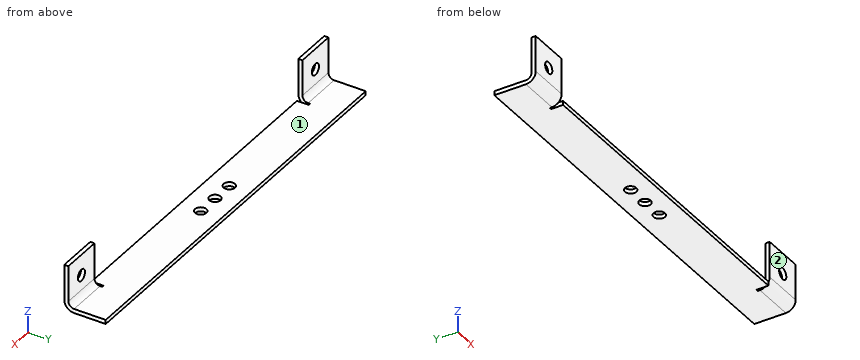
```python
from build123d import *

# Parameters (mm, degrees)
SKETCH_1_W                        = 200
SKETCH_1_H                        = 20
SM_BASE_FLANGE_1_DEPTH            = 2
SM_EDGE_FLANGE_1_STRIP_W          = 13.4732
SM_EDGE_FLANGE_1_STRIP_H          = 2
SM_EDGE_FLANGE_1_STRIP_CUT_DEPTH  = 20
SM_EDGE_FLANGE_1_RELIEF_W         = 14.4732
SM_EDGE_FLANGE_1_RELIEF_H         = 1
SM_EDGE_FLANGE_1_RELIEF_CUT_DEPTH = 2
SM_EDGE_FLANGE_1_DEPTH            = 20
SKETCH_10_R                       = 2.75
CUT_EXTRUDE_2_DEPTH               = 10
SKETCH_11_R                       = 2.75
CUT_EXTRUDE_3_DEPTH               = 10


# Sheet-metal steps are written as plain solids
with BuildPart() as part:
    # Sketch 1 → 基体-法兰1 (new body)
    with BuildSketch(Plane.XY):
        with Locations((0, -10)):
            Rectangle(SKETCH_1_W, SKETCH_1_H)
    extrude(amount=-SM_BASE_FLANGE_1_DEPTH)

    # 边线-法兰1 strip (across the edge) → 边线-法兰1 strip cut (cut)
    with BuildSketch(Plane(origin=(-100, -20, 0), x_dir=(0, 1, 0), z_dir=(1, 0, 0))):
        with Locations((-2, -1)):
            Rectangle(SM_EDGE_FLANGE_1_STRIP_W, SM_EDGE_FLANGE_1_STRIP_H)
    sm_edge_flange_1_strip_cut = extrude(amount=SM_EDGE_FLANGE_1_STRIP_CUT_DEPTH, mode=Mode.SUBTRACT)

    # 边线-法兰1 relief (on the sheet) → 边线-法兰1 relief cut (cut)
    with BuildSketch(Plane(origin=(-100, -15.2634, 0), x_dir=(0, 1, 0), z_dir=(0, 0, 1))):
        with Locations((-6.2366, -20.5)):
            Rectangle(SM_EDGE_FLANGE_1_RELIEF_W, SM_EDGE_FLANGE_1_RELIEF_H)
    sm_edge_flange_1_relief_cut = extrude(amount=-SM_EDGE_FLANGE_1_RELIEF_CUT_DEPTH, mode=Mode.SUBTRACT)

    # 边线-法兰1 section (across the edge) → 边线-法兰1 (add)
    with BuildSketch(Plane(origin=(-100, -20, 0), x_dir=(0, 1, 0), z_dir=(1, 0, 0))):
        with BuildLine():
            Line((0, 2.7366), (0, 20))
            Line((0, 20), (2, 20))
            Line((2, 20), (2, 2.7366))
            ThreePointArc((2, 2.7366), (2.801531583, 0.801531583), (4.7366, 0))
            Line((4.7366, 0), (4.7366, -2))
            ThreePointArc((4.7366, -2), (1.38731802, -0.61268198), (0, 2.7366))
        make_face()
    sm_edge_flange_1 = extrude(amount=SM_EDGE_FLANGE_1_DEPTH)

    # 草图10 → 切除-拉伸2 (cut)
    with BuildSketch(Plane(origin=(0, -18, 0), x_dir=(1, 0, 0), z_dir=(0, 1, 0))):
        with Locations(Location((-90, -10, 0), (0, 0, 270))):
            Circle(SKETCH_10_R)
    cut_extrude_2 = extrude(amount=-CUT_EXTRUDE_2_DEPTH, mode=Mode.SUBTRACT)

    # 镜向1: 边线-法兰1 strip cut, 边线-法兰1 relief cut, 边线-法兰1, 切除-拉伸2 across plane
    add(sm_edge_flange_1_strip_cut.mirror(Plane(origin=(0, 0, 0), x_dir=(0, 0, 1), z_dir=(1, 0, 0))), mode=Mode.SUBTRACT)
    add(sm_edge_flange_1_relief_cut.mirror(Plane(origin=(0, 0, 0), x_dir=(0, 0, 1), z_dir=(1, 0, 0))), mode=Mode.SUBTRACT)
    add(sm_edge_flange_1.mirror(Plane(origin=(0, 0, 0), x_dir=(0, 0, 1), z_dir=(1, 0, 0))))
    add(cut_extrude_2.mirror(Plane(origin=(0, 0, 0), x_dir=(0, 0, 1), z_dir=(1, 0, 0))), mode=Mode.SUBTRACT)

    # 草图11 → 切除-拉伸3 (cut)
    with BuildSketch(Plane(origin=(0, 0, -2), x_dir=(-1, 0, 0), z_dir=(0, 0, -1))):
        with Locations((0, -10)):
            Circle(SKETCH_11_R)
        with Locations((-11, -10)):
            Circle(SKETCH_11_R)
        with Locations(Location((11, -10, 0), (0, 0, 180))):
            Circle(SKETCH_11_R)
    extrude(amount=-CUT_EXTRUDE_3_DEPTH, mode=Mode.SUBTRACT)


solid = part.part
```
The listing builds one solid part. Answer for the finished solid, in the listing's coordinates (mm). Face numbers are marked on the shaded views. Give positions to 0.01 mm unless a question says otherwise; leave off trailing zeros. Order: outer loops, then holes, each group sorted by start corner. A loop starts at its lowest first (then second) coordinate and runs counter-clockwise, first axis right, second up.
Item 1: For a pull along X with two mould halves and no side action, classify the marked faces 1 and 2 as pulls with the +X half, pulls with the -X half, needs draft (parallel to the pull), parting line crosses it, or undercut.
From the geometry:
face 1: undercut
face 2: needs draft
Item 2: Given pin 1 Ø6 at (x, y) = (7.5, -8.5) entering from +Z; pin 2 Ø3.5 at (x, z) = (-90, 10) entering from -Y; pin 3 Ø1.1 at (x, z) = (-79.5, -1) entering from -Y; pin 4 Ø5 at (x, z) = (90.5, 9.5) entering from +Y, each flat-ended and moving along its own axis, determine where each tip first touches the part or whether it passes through.
From the geometry:
pin 1: stops at z = 0
pin 2: passes through
pin 3: stops at y = -20
pin 4: stops at y = -18
Item 3: The part is cut by section B-B, the plane y = -10. Give the vertices of the cut face in (x, z).
From the geometry:
outline: (-100, -2) - (-13.75, -2) - (-13.75, 0) - (-100, 0) - close; (-8.25, -2) - (-2.75, -2) - (-2.75, 0) - (-8.25, 0) - close; (2.75, -2) - (8.25, -2) - (8.25, 0) - (2.75, 0) - close; (13.75, -2) - (100, -2) - (100, 0) - (13.75, 0) - close
Item 4: The part is cut by section A-A, the plane x = -90. Give the vertices of the cut face in (y, z).
From the geometry:
outline: (-20, 2.74) arc R4.74 ccw to (-15.26, -2) - (0, -2) - (0, 0) - (-15.26, 0) arc R2.74 cw to (-18, 2.74) - (-18, 7.25) - (-20, 7.25) - close; (-20, 12.75) - (-18, 12.75) - (-18, 20) - (-20, 20) - close
Item 5: The part is cut by section D-D, the plane x = -11. Give the vertices of the cut face in (y, z).
From the geometry:
outline: (-20, -2) - (-12.75, -2) - (-12.75, 0) - (-20, 0) - close; (-7.25, -2) - (0, -2) - (0, 0) - (-7.25, 0) - close
Item 6: Find the intervals of material crossed by probe 1 along X at (y, z) = (-18.45, 10); probe 2 along X at (y, z) = (-19, 7.75); probe 3 along Z at (x, y) = (70, -9), in increasing order.
From the geometry:
probe 1: x = -100 to -92.75, -87.25 to -80, 80 to 87.25, 92.75 to 100
probe 2: x = -100 to -91.58, -88.42 to -80, 80 to 88.42, 91.58 to 100
probe 3: z = -2 to 0
Item 7: The part is cut by section C-C, the plane z = 10. Give the vertices of the cut face in (x, y).
From the geometry:
outline: (-100, -20) - (-92.75, -20) - (-92.75, -18) - (-100, -18) - close; (-87.25, -20) - (-80, -20) - (-80, -18) - (-87.25, -18) - close; (80, -20) - (87.25, -20) - (87.25, -18) - (80, -18) - close; (92.75, -20) - (100, -20) - (100, -18) - (92.75, -18) - close
